from build123d import *

# Parameters (mm, degrees)
F2_R      = 1.5875
F3_DEPTH  = 7.501
F5_DEPTH  = 9.5
F6_R      = 2
F7_DEPTH  = 16.501
F9_R      = 3.75
F10_DEPTH = 5


with BuildPart() as f1:
    # F0 (on Front) → F1 (revolve)
    with BuildSketch(Plane.XZ):
        with BuildLine():
            Line((0, 17.5), (0, 0))
            Line((0, 0), (4, 0))
            Line((4, 0), (4, 9))
            Line((4, 9), (7.5, 9))
            Line((7.5, 9), (7.5, 17.5))
            Line((7.5, 17.5), (6.13125, 17.5))
            Line((6.13125, 17.5), (6.13125, 15.08125))
            ThreePointArc((6.13125, 15.08125), (3.75, 12.7), (1.36875, 15.08125))
            Line((1.36875, 15.08125), (1.36875, 17.5))
            Line((1.36875, 17.5), (0, 17.5))
        make_face()
    revolve(axis=Axis((2, 0, 0), (-1, 0, 0)))

    # F2 (on face) → F3 (cut, through all)
    with BuildSketch(Plane.YZ.offset(7.5)):
        Circle(F2_R)
    extrude(amount=-F3_DEPTH, mode=Mode.SUBTRACT)

    # F4 (on face) → F5 (join)
    with BuildSketch(Plane(origin=(0, 0, 0), x_dir=(0, -1, 0), z_dir=(-1, 0, 0))):
        with BuildLine():
            Line((-1.2329461667, -1), (-10.9544511501, -1))
            ThreePointArc((-10.9544511501, -1), (0, -11), (10.9544511501, -1))
            Line((10.9544511501, -1), (1.2329461667, -1))
            ThreePointArc((1.2329461667, -1), (0, -1.5875), (-1.2329461667, -1))
        make_face()
    extrude(amount=F5_DEPTH)

    # F6 (on face) → F7 (cut, through all)
    with BuildSketch(Plane.XY.offset(-1)):
        with Locations((-5.25, 6.5)):
            Circle(F6_R)
        with Locations((-5.25, -6.5)):
            Circle(F6_R)
    extrude(amount=-F7_DEPTH, mode=Mode.SUBTRACT)

    # F9 (on offset) → F10 (cut)
    with BuildSketch(Plane.XY.offset(-11)):
        with Locations((-5.25, -6.5)):
            Circle(F9_R)
    extrude(amount=F10_DEPTH, mode=Mode.SUBTRACT)


solid = f1.part
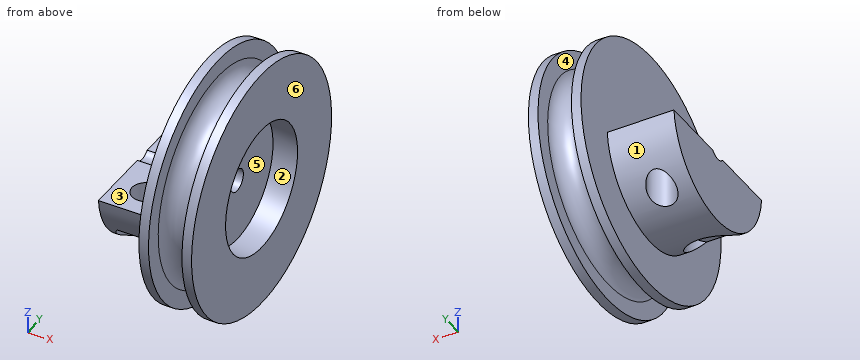
Geometry: final body of the model. Coordinates: model frame, mm. Face numbers are marked on the shaded views. A direction names the side the tool comes from. Give positions to 0.01 mm unless a question says otherwise; leave off trailing zeros. Loops run counter-clockwise (first coordinate to the right, second up) from the corner with the lowest first, then second, coordinate; pieces in that order, holes last. Notation, with made-up numbers: (-11, -21.75) - (16, -21.75) arc R28 ccw to (16, 5.25) - close; hole circle Ø11 at (73, 44.5). An arc over 180 degrees is marked (long way). Answer as CSV lines item,"result". Start each with the question number.
1. Pin query (flat end, axial travel): P1, Ø3, axis at x = -4.5, y = -5, coming from the +Z side; P2, Ø8, axis at x = 4, z = 7.5, coming from the +Y side; P3, Ø6, axis at x = 4, z = 6, coming from the +Y side; P4, Ø14.5, axis at y = 3, z = 2.5, coming from the +X side. Return the tip coordinate at first contact, or that it passes through.
2. Ray query, L1, parallel to X at y = -15, z = -8; L2, parallel to X at y = 6.5, z = -5.25; L3, parallel to Y at x = -5.25, z = -4.05. Return the intervals inside material, ascending.
3. Draft query along Y for the marked faces 1, 2 and 3. Return one class per face: released by +Y, released by -Y, zero draft, split by the parting line, or undercut.
4. Section A-A, the plane y = 0. Return loops of the section in (x, z), plus the area to 3 significant figures.
5. Reachability of the marked faces 4, 5 and 6 from +Z, -Z, +X, -X, +Y, -Y: full face, straight path, thin tool, end or side. Return the list, or none.
6. Section C-C, the plane x = -5.25. Give the number of separate pieces and of enclosed holes in the cut face, plus the area to 3 significant figures.
7. Section B-B, the plane z = 0. Return loops of the section in (x, y), plus the area to 3 significant figures.
Answers:
1,P1,"stops at z = -1"
1,P2,"stops at y = 17.01"
1,P3,"stops at y = 17.06"
1,P4,"stops at x = 7.5"
2,L1,"x = 0 to 1.37, 6.13 to 7.5"
2,L2,"x = -9.5 to -7.25, -3.25 to 4"
2,L3,"y = -10.23 to -8.5, -4.5 to 4.5, 8.5 to 10.23"
3,face 1,"split by the parting line"
3,face 2,"undercut"
3,face 3,"zero draft"
4,outline,"(-9.5, -11) - (0, -11) - (0, -17.5) - (1.37, -17.5) - (1.37, -15.08) arc R2.38 cw to (6.13, -15.08) - (6.13, -17.5) - (7.5, -17.5) - (7.5, -9) - (4, -9) - (4, -1.59) - (-9.5, -1.59) - close; (0, 1.59) - (4, 1.59) - (4, 9) - (7.5, 9) - (7.5, 17.5) - (6.13, 17.5) - (6.13, 15.08) arc R2.38 cw to (1.37, 15.08) - (1.37, 17.5) - (0, 17.5) - close"
4,area,"235 mm2"
5,face 4,"none"
5,face 5,"+X"
5,face 6,"+Z, -Z, +X, +Y, -Y"
6,separate pieces,"3"
6,enclosed holes,"0"
6,area,"97.0 mm2"
7,outline,"(0, -17.5) - (1.37, -17.5) - (1.37, -15.08) arc R2.38 cw to (6.13, -15.08) - (6.13, -17.5) - (7.5, -17.5) - (7.5, -9) - (4, -9) - (4, -1.59) - (0, -1.59) - close; (0, 1.59) - (4, 1.59) - (4, 9) - (7.5, 9) - (7.5, 17.5) - (6.13, 17.5) - (6.13, 15.08) arc R2.38 cw to (1.37, 15.08) - (1.37, 17.5) - (0, 17.5) - close"
7,area,"146 mm2"
